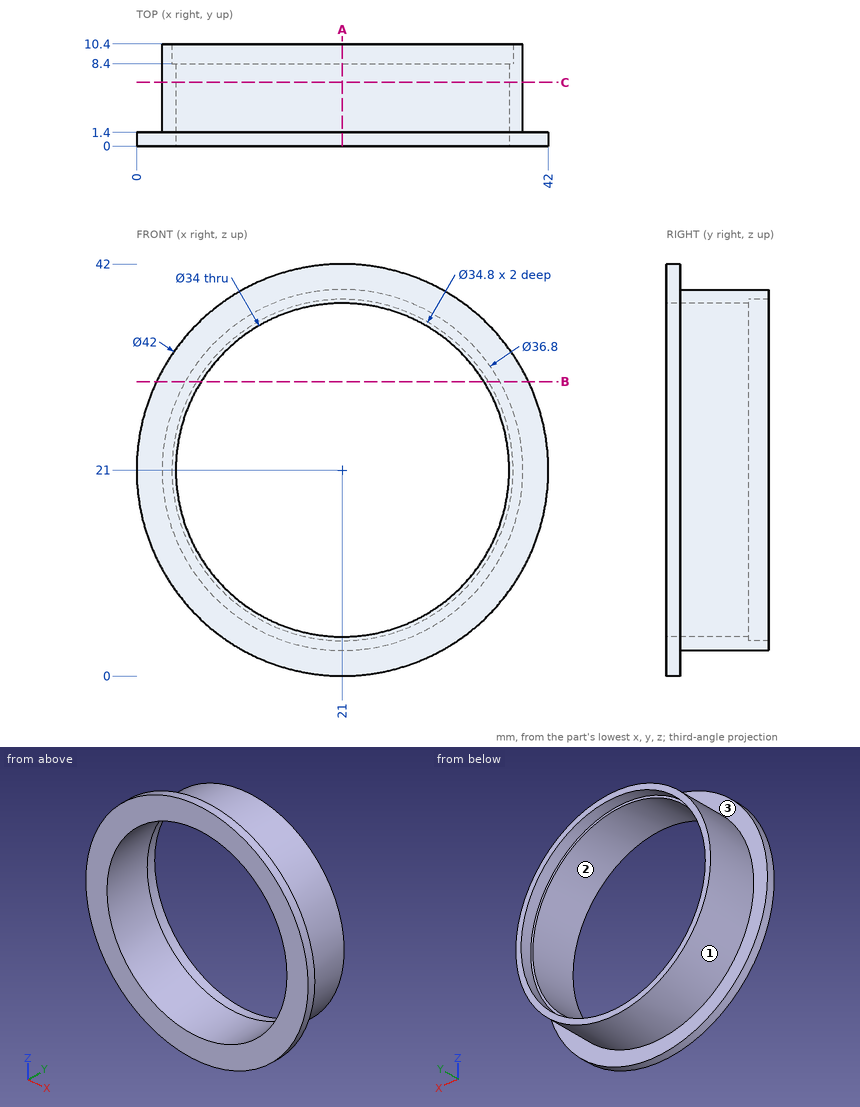
Here's the drawing with two shaded views (mm, measured from the low corner). I have some questions. Coordinates: 2 decimals unless noted, no trailing zeros. Order: outer loops, then holes, each group sorted by start corner. A loop starts at its lowest first (then second) coordinate and runs counter-clockwise, first axis right, second up. Notation, with made-up numbers: (58, 65.5) -> (78, 65.5) arc R29 cw to (78, 87.5) -> close; hole circle Ø7 at (39.25, 73). An arc over 180 degrees is marked (long way). One line per question, with ' | ' between items.
Q1. Imagine slicing it at A-A on x = 21. Please give me the cut outline in (y, z).
Return value:
outline: (0, 0) -> (1.4, 0) -> (1.4, 2.6) -> (10.4, 2.6) -> (10.4, 3.6) -> (8.4, 3.6) -> (8.4, 4) -> (0, 4) -> close; (0, 38) -> (8.4, 38) -> (8.4, 38.4) -> (10.4, 38.4) -> (10.4, 39.4) -> (1.4, 39.4) -> (1.4, 42) -> (0, 42) -> close
Q2. If I drill on L1, parallel to X at y = 7.75, z = 20.5; L2, parallel to Z at x = 21, y = 9.1, over which ranges is the centre line in solid material (lowest first)?
Return value:
L1: 2.61 to 4.01, 37.99 to 39.39 | L2: 2.6 to 3.6, 38.4 to 39.4
Q3. Thinking about a two-plate mould opening in X: for the marked faces 1, 2 and 3, which applies, pulls with the +X half, pulls with the -X half, needs draft (parallel to the pull), parting line crosses it, or undercut?
Return value:
face 1: parting line crosses it | face 2: undercut | face 3: needs draft
Q4. I'm going to push flat-ended pins straight in: P1, Ø1, axis at y = 3.5, z = 29, coming from the +X side; P2, Ø1.5, axis at x = 12, z = 8, coming from the +Y side; P3, Ø6, axis at x = 13, y = 4.5, coming from the -Z side; P4, Ø2, axis at y = 6, z = 19, coming from the -X side. Where does each tip first touch, or does it pass through?
Return value:
P1: x = 37.8 | P2: through | P3: z = 3.29 | P4: x = 2.63
Q5. Imagine slicing it at B-B on z = 30. Please give me the cut outline in (x, y), and give its area (3 significant figures).
Return value:
outline: (2.03, 0) -> (6.58, 0) -> (6.58, 8.4) -> (6.11, 8.4) -> (6.11, 10.4) -> (4.95, 10.4) -> (4.95, 1.4) -> (2.03, 1.4) -> close; (35.42, 0) -> (39.97, 0) -> (39.97, 1.4) -> (37.05, 1.4) -> (37.05, 10.4) -> (35.89, 10.4) -> (35.89, 8.4) -> (35.42, 8.4) -> close | area: 40.1 mm²
Q6. Imagine slicing it at C-C on y = 6.5. Please give me the cut outline in (x, z), and give its area (3 significant figures).
Return value:
outline: circle Ø36.8 at (21, 21); hole circle Ø34 at (21, 21) | area: 156 mm²
